Source: CAD feature listing. Evaluate the final solid. Frame: model axes, mm. Face numbers are marked on the shaded views. A direction names the side the tool comes from. Round coordinates to 2 decimals unless told otherwise and drop trailing zeros. Write each loop counter-clockwise with the first axis right and the second up, starting at its lowest first coordinate (ties: lowest second). Pieces come first, ordered by that corner, then holes.
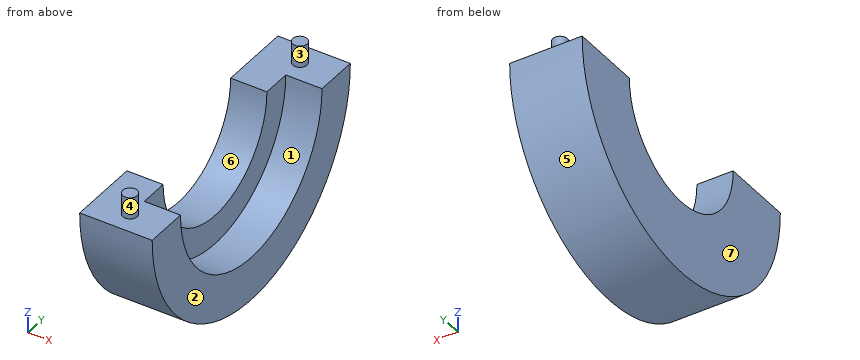
```python
from build123d import *

# Parameters (mm, degrees)
REVOLVE1_ANGLE      = 180
SKETCH2_R           = 0.5
BOSS_EXTRUDE1_DEPTH = 1.5


with BuildPart() as part:
    # Sketch1 → Revolve1 (revolve)
    with BuildSketch(Plane.XY):
        Polygon((-2.5, 5.5), (-5, 5.5), (-5, 10.5), (0, 10.5), (0, 7.5), (-2.5, 7.5), align=None)
    revolve(axis=Axis((0, 0, 0), (-1, 0, 0)), revolution_arc=REVOLVE1_ANGLE)

    # Sketch2 → Boss-Extrude1 (add)
    with BuildSketch(Plane.XY):
        with Locations((-2.5, 9)):
            Circle(SKETCH2_R)
    boss_extrude1 = extrude(amount=BOSS_EXTRUDE1_DEPTH)

    # Mirror1: Boss-Extrude1 across plane
    add(boss_extrude1.mirror(Plane.ZX))


solid = part.part
```
Q1. Mould query, pull axis Y, two halves, no side actions, for the marked faces 4, 5, 6 and 7. Classes: pulls with the +Y half, pulls with the -Y half, needs draft (parallel to the pull), parting line crosses it, or undercut.
Q2. Section query A-A, the plane z = -2.25. Output: boundary loops of the cut face in (x, y).
Q3. Set-up query: the marked faces 1, 2 and 3. Return all of +Z, -Z, +X, -X, +Y, -Y with unobstructed straight access to the full face (end or side cutting, diameter ignored); none if empty.
Q4. Section query B-B, the plane y = 0. Output: boundary loops of the cut face in (x, z).
Q5. Section query D-D, the plane z = -5.75. Output: boundary loops of the cut face in (x, y), and give its area (3 significant figures).
Q6. Pin query (flat end, axial travel): P1, Ø1.5, axis at x = -2, z = -7.5, coming from the +Y side; P2, Ø3, axis at x = -2, z = -5.5, coming from the +Y side; P3, Ø1, axis at x = -1, y = 4.5, coming from the -Z side. Return the tip coordinate at first contact, or that it passes through.
Q7. Section query C-C, the plane x = -2.7. Output: boundary loops of the cut face in (y, z).
Q8. Line query: line 1 (Y direction, x = -3.3, z = -2.25); line 2 (Y direction, x = -3.3, z = -3.5); line 3 (X direction, y = -4.75, z = -3.25). Output: solid intervals per line, ascending.
Filled in:
1. face 4: undercut
1. face 5: parting line crosses it
1. face 6: undercut
1. face 7: needs draft
2. outline: (-5, -10.26) - (0, -10.26) - (0, -7.15) - (-2.5, -7.15) - (-2.5, -5.02) - (-5, -5.02) - close; (-5, 5.02) - (-2.5, 5.02) - (-2.5, 7.15) - (0, 7.15) - (0, 10.26) - (-5, 10.26) - close
3. face 1: +Z, +X
3. face 2: +Z, -Z, +X, +Y, -Y
3. face 3: +Z
4. outline: (-5, -10.5) - (0, -10.5) - (0, -7.5) - (-2.5, -7.5) - (-2.5, -5.5) - (-5, -5.5) - close
5. outline: (-5, -8.79) - (0, -8.79) - (0, -4.82) - (-2.5, -4.82) - (-2.5, 4.82) - (0, 4.82) - (0, 8.79) - (-5, 8.79) - close
5. area: 63.8 mm2
6. P1: stops at y = 8.04
6. P2: stops at y = 9.71
6. P3: stops at z = -9.71
7. outline: (-10.5, 0) arc R10.5 ccw to (10.5, 0) - (9.46, 0) - (9.46, 1.5) - (8.54, 1.5) - (8.54, 0) - (5.5, 0) arc R5.5 cw to (-5.5, 0) - (-8.54, 0) - (-8.54, 1.5) - (-9.46, 1.5) - (-9.46, 0) - close
8. line 1: y = -10.26 to -5.02, 5.02 to 10.26
8. line 2: y = -9.9 to -4.24, 4.24 to 9.9
8. line 3: x = -5 to -2.5
